Source: CAD feature listing. Evaluate the final solid. Frame: model axes, mm. A direction names the side the tool comes from. Round coordinates to 2 decimals unless told otherwise and drop trailing zeros. Loops run counter-clockwise (first coordinate to the right, second up) from the corner with the lowest first, then second, coordinate; pieces in that order, holes last.
(1) Section A-A, the plane y = 0. Return the cut outline in (x, z).
(2) Section C-C, the plane x = 10. Return the cut outline in (y, z), plus the area to 3 significant figures.
(3) First-contact query: pin 1 Ø5 at (x, z) = (12, -3) entering from -Y; pin 2 Ø2 at (x, y) = (1, 3) entering from -Z; pin 3 Ø1 at (x, z) = (23, 0.5) entering from +Y. Flat tips, straight axial feed; report the tip coordinate or a pass-through.
(4) Set-up query: faces 1 (the flat face through (0, 4, 4)), 2 (the flat face through (21.5, -4, -7)), 3 (the flat face through (60, 0, 0)). Return all of +Z, -Z, +X, -X, +Y, -Y with unobstructed straight access to the full face (end or side cutting, diameter ignored); none if empty.
(5) Material intervals for probe 1 along X at (y, z) = (-6.5, -1); probe 2 along X at (y, z) = (4.5, -1); probe 3 along Y at (x, z) = (1, 0.25), sorted ascending.
(6) Section D-D, the plane x = 25. Return the cut outline in (y, z), plus the area to 3 significant figures.
```python
from build123d import *


with BuildPart() as part:
    # Sketch1 → Revolve1 (revolve)
    with BuildSketch(Plane.XY, mode=Mode.PRIVATE) as revolve1_sk:
        with BuildLine():
            Line((-1, 5), (-28, 5))
            Line((-28, 5), (-28, 0))
            Line((-28, 0), (60, 0))
            Line((60, 0), (60, 7.5))
            Line((60, 7.5), (21.7, 7.5))
            ThreePointArc((21.7, 7.5), (21.558578644, 7.558578644), (21.5, 7.7))
            Line((21.5, 7.7), (21.5, 9))
            Line((21.5, 9), (0, 9))
            Line((0, 9), (0, 5))
            ThreePointArc((0, 5), (-0.5, 4.5), (-1, 5))
        make_face()
    revolve(revolve1_sk.sketch.rotate(Axis((-49.812651096, 0, 0), (1, 0, 0)), 90), axis=Axis((-49.812651096, 0, 0), (1, 0, 0)))  # turned: the seam where the file's is


solid = part.part
```
Output values:
1. outline: (-28, -5) - (-1, -5) arc R0.5 cw to (0, -5) - (0, -9) - (21.5, -9) - (21.5, -7.7) arc R0.2 cw to (21.7, -7.5) - (60, -7.5) - (60, 7.5) - (21.7, 7.5) arc R0.2 cw to (21.5, 7.7) - (21.5, 9) - (0, 9) - (0, 5) arc R0.5 cw to (-1, 5) - (-28, 5) - close
2. outline: circle Ø18 at (0, 0)
2. area: 254 mm2
3. pin 1: stops at y = -8.99
3. pin 2: stops at z = -8.77
3. pin 3: stops at y = 7.5
4. face 1: -X
4. face 2: +X
4. face 3: +Z, -Z, +X, +Y, -Y
5. probe 1: x = 0 to 60
5. probe 2: x = -28 to -0.81, -0.19 to 60
5. probe 3: y = -9 to 9
6. outline: circle Ø15 at (0, 0)
6. area: 177 mm2
